Part model, mm, in its own coordinate system. Face numbers are marked on the shaded views. A direction names the side the tool comes from. Round coordinates to 2 decimals unless told otherwise and drop trailing zeros. Write each loop counter-clockwise with the first axis right and the second up, starting at its lowest first coordinate (ties: lowest second). Pieces come first, ordered by that corner, then holes. Notation, with made-up numbers: M 18,22.5 L 72,22.5 A28 cw 72,50.5 Z; hole C 77.25,-38.75 d4. An arc over 180 degrees is marked long. Use a Markdown table: item, result. Add a question column.
1) Two-plate mould, pull along X, no slides. Class the marked faces 1, 2 and 3: released by +X, released by -X, zero draft, split by the parting line, or undercut.
2) Wall check: probe 1 along X at (y, z) = (49.5, -1.8); probe 2 along X at (y, z) = (48, -3.1); probe 3 along Y at (x, z) = (-72.5, -0.75). Give the ranges that are in metal, low to high.
3) Drop a flat-ended pin along its axis: P1, Ø4, axis at x = -51.54, y = 47.72, coming from the +Z side. Give the stop position or say it passes through.
4) Slice it at A-A on x = -74.5. Write the cut outline in (y, z), plus the area to 3 significant figures.
5) Slice it at D-D on x = -49.5. Write the cut outline in (y, z), plus the area to 3 significant figures.
6) Slice it at C-C on z = -1.75. Write the cut outline in (x, y) (3 decimals).
7) Which spindle directions (+Z, -Z, +X, -X, +Y, -Y) get a long thin tool onto all of the face, cutting with end or side? Do the marked faces 4 and 5. Say none if no direction does.
8) Slice it at B-B on y = 58. Write the cut outline in (x, z), plus the area to 3 significant figures.
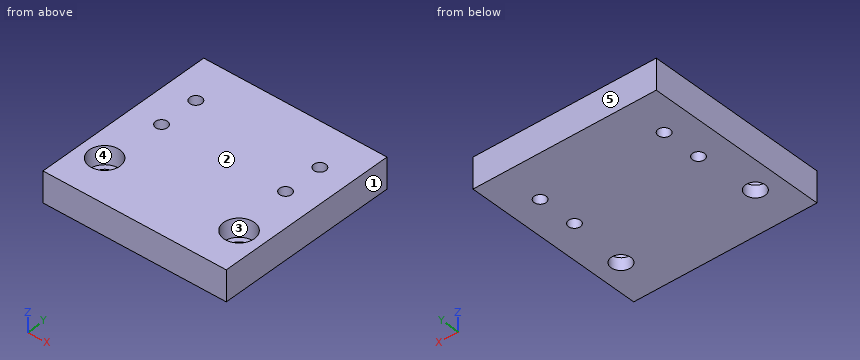
```python
from build123d import *

# Parameters (mm, degrees)
F0_W           = 30
F0_H           = 30
F1_DEPTH       = 5
F3_D           = 3.2
F3_CBORE_D     = 5
F3_CBORE_DEPTH = 3
F4_D           = 1.95


with BuildPart() as f1:
    # F0 (on Top) → F1 (new body)
    with BuildSketch(Plane.XY):
        with Locations((-62.535277, 55.776885)):
            Rectangle(F0_W, F0_H)
    extrude(amount=-F1_DEPTH)

    # F3 (through all)
    with Locations(Plane.XY):
        with Locations((-73.535277, 47.719706), (-51.535277, 47.719706)):
            CounterBoreHole(F3_D / 2, F3_CBORE_D / 2, F3_CBORE_DEPTH)

    # F4 (through all)
    with Locations(Plane.XY):
        with Locations((-52.385277, 57.376885), (-52.385277, 63.776885), (-72.685277, 57.376885), (-72.685277, 63.776885)):
            Hole(F4_D / 2)


solid = f1.part
```
Entries:
| question | item | result |
|---|---|---|
| 1 | face 1 | released by +X |
| 1 | face 2 | zero draft |
| 1 | face 3 | undercut |
| 2 | probe 1 | x = -77.54 to -75.29, -71.78 to -53.29, -49.78 to -47.54 |
| 2 | probe 2 | x = -77.54 to -75.11, -71.96 to -53.11, -49.96 to -47.54 |
| 2 | probe 3 | y = 40.78 to 45.44, 50 to 56.42, 58.33 to 62.82, 64.73 to 70.78 |
| 3 | P1 | stops at z = -3 |
| 4 | outline | M 40.78,-5 L 46.44,-5 L 46.44,-3 L 45.41,-3 L 45.41,0 L 40.78,0 Z; M 49,-5 L 70.78,-5 L 70.78,0 L 50.03,0 L 50.03,-3 L 49,-3 Z |
| 4 | area | 131 mm^2 |
| 5 | outline | M 40.78,-5 L 70.78,-5 L 70.78,0 L 49.17,0 L 49.17,-3 L 46.27,-3 L 46.27,0 L 40.78,0 Z |
| 5 | area | 141 mm^2 |
| 6 | outline | M -77.535,40.777 L -47.535,40.777 L -47.535,70.777 L -77.535,70.777 Z; hole C -73.535,47.72 d5; hole C -72.685,57.377 d1.95; hole C -72.685,63.777 d1.95; hole C -51.535,47.72 d5; hole C -52.385,57.377 d1.95; hole C -52.385,63.777 d1.95 |
| 7 | face 4 | +Z |
| 7 | face 5 | +Z, -Z, +X, -X, +Y |
| 8 | outline | M -77.54,-5 L -73.44,-5 L -73.44,0 L -77.54,0 Z; M -71.94,-5 L -53.14,-5 L -53.14,0 L -71.94,0 Z; M -51.64,-5 L -47.54,-5 L -47.54,0 L -51.64,0 Z |
| 8 | area | 135 mm^2 |
